```python
from build123d import *

# Parameters (mm, degrees)
EXTRUDE_1_DEPTH     = 2
SKETCH_2_W          = 6
SKETCH_2_H          = 12
EXTRUDE_2_DEPTH     = 5
FILLET_1_RADIUS     = 3
FILLET_1_LENGTH     = 10
SKETCH_4_R          = 1.1
CUT_EXTRUDE_2_DEPTH = 28
SKETCH_7_R          = 1.1
CUT_EXTRUDE_5_DEPTH = 3.5
SKETCH_9_R          = 1.5
CUT_EXTRUDE_7_DEPTH = 0.1
SKETCH_15_W         = 6
SKETCH_15_H         = 9.205828816
CUT_EXTRUDE_8_DEPTH = 10


with BuildPart() as part:
    # 草图1 → 凸台-拉伸1 (new body)
    with BuildSketch(Plane(origin=(0, 0, 0), x_dir=(1, 0, 0), z_dir=(0, 1, 0))):
        with BuildLine():
            Line((-7, 3), (7, 3))
            ThreePointArc((7, 3), (10, 0), (7, -3))
            Line((7, -3), (-7, -3))
            ThreePointArc((-7, -3), (-10, 0), (-7, 3))
        make_face()
    extrude(amount=EXTRUDE_1_DEPTH)

    # 草图2 → 凸台-拉伸2 (add, symmetric)
    with BuildSketch(Plane(origin=(0, 0, 0), x_dir=(0, 0, -1), z_dir=(1, 0, 0))):
        with Locations((0, 6)):
            Rectangle(SKETCH_2_W, SKETCH_2_H)
    extrude(amount=EXTRUDE_2_DEPTH, both=True)

    # 圆角1: full round fillet: the end face becomes a half cylinder, R = half its width
    fillet_1_face = Plane((0, 12, 0), x_dir=(1, 0, 0), z_dir=(0, 1, 0))  # on the end face: x along it, z out of the body
    fillet_1_slab = fillet_1_face.offset(-FILLET_1_RADIUS / 2) * Box(FILLET_1_LENGTH, 2 * FILLET_1_RADIUS, FILLET_1_RADIUS, mode=Mode.PRIVATE)  # the body's end, R deep
    fillet_1_round = Plane((0, 9, 0), x_dir=(0, 1, 0), z_dir=(1, 0, 0)) * Cylinder(FILLET_1_RADIUS, FILLET_1_LENGTH, mode=Mode.PRIVATE)  # its axis R under the face
    add(fillet_1_slab - fillet_1_round, mode=Mode.SUBTRACT)

    # 草图4 → 切除-拉伸2 (cut)
    with BuildSketch(Plane(origin=(5, 0, 0), x_dir=(0, 0, -1), z_dir=(1, 0, 0))):
        with Locations((0, 9)):
            Circle(SKETCH_4_R)
    extrude(amount=-CUT_EXTRUDE_2_DEPTH, mode=Mode.SUBTRACT)

    # 草图7 → 切除-拉伸5 (cut)
    with BuildSketch(Plane(origin=(0, 2, 0), x_dir=(1, 0, 0), z_dir=(0, 1, 0))):
        with Locations(Location((7, 0, 0), (0, 0, 270))):
            Circle(SKETCH_7_R)
        with Locations(Location((-7, 0, 0), (0, 0, 270))):
            Circle(SKETCH_7_R)
    extrude(amount=-CUT_EXTRUDE_5_DEPTH, mode=Mode.SUBTRACT)

    # 草图9 → 切除-拉伸7 (cut)
    with BuildSketch(Plane.XZ):
        with Locations(Location((0, 0, 0), (0, 0, 270))):
            Circle(SKETCH_9_R)
    extrude(amount=-CUT_EXTRUDE_7_DEPTH, mode=Mode.SUBTRACT)

    # 草图15 → 切除-拉伸8 (cut)
    with BuildSketch(Plane(origin=(0, 0, -3), x_dir=(-1, 0, 0), z_dir=(0, 0, -1))):
        with Locations((0, 9.102914408)):
            Rectangle(SKETCH_15_W, SKETCH_15_H)
    extrude(amount=-CUT_EXTRUDE_8_DEPTH, mode=Mode.SUBTRACT)


solid = part.part
```
Verification items for the finished model (mm, model axes). A direction names the side the tool comes from. Coordinates: 2 decimals unless noted, no trailing zeros. Order: outer loops, then holes, each group sorted by start corner. A loop starts at its lowest first (then second) coordinate and runs counter-clockwise, first axis right, second up. Notation, with made-up numbers: (-34.75, 25) - (-9.75, 25) arc R21 cw to (-9.75, 40) - close; hole circle Ø11 at (83, 12.25). An arc over 180 degrees is marked (long way). Return JSON: item names as keys, results as strings.
(1) Section check B-B, the plane z = 0. Give the number of separate pieces and of enclosed holes in the cut face, and give its area (3 significant figures).
Filled sheet:
{"separate pieces": "5", "enclosed holes": "0", "area": "77.1 mm^2"}
(2) Thickness scan on line 1 along X through (y, z) = (1.2, 0); line 2 along Y through (x, z) = (-4.25, 0.05); line 3 along X through (y, z) = (10.5, -2.4). Record the ranges inside material, lowest first.
Filled sheet:
{"line 1": "x = -10 to -8.1, -5.9 to 5.9, 8.1 to 10", "line 2": "y = 0 to 7.9, 10.1 to 12", "line 3": "x = -5 to -3, 3 to 5"}
(3) Section check D-D, the plane x = 6.75. Record the cut outline in (y, z), and give its area (3 significant figures).
Filled sheet:
{"outline": "(0, -3) - (2, -3) - (2, -1.07) - (0, -1.07) - close; (0, 1.07) - (2, 1.07) - (2, 3) - (0, 3) - close", "area": "7.72 mm^2"}
(4) Section check A-A, the plane y = 5. Record the cut outline in (x, z).
Filled sheet:
{"outline": "(-5, -3) - (-3, -3) - (-3, 3) - (-5, 3) - close; (3, -3) - (5, -3) - (5, 3) - (3, 3) - close"}
(5) Access from +Z, -Z, +X, -X, +Y, -Y to the whole of each face (thin tool, end or side, straight path). Record for faces 1 (the flat face through (0, 0.1, 0)), 2 (the flat face through (-8, 2, 1)), 3 (the flat face through (8, 2, 1)), 4 (the flat face through (3, 7, 0)), 5 (the cylindrical face through (-10, 1, 0)).
Filled sheet:
{"face 1": "-Y", "face 2": "+Z, -Z, -X, +Y", "face 3": "+Z, -Z, +X, +Y", "face 4": "+Z, -Z, +Y", "face 5": "-X, +Y, -Y"}
(6) Go/stop test with flat-tipped pins: pin 1 (1.8 mm diameter, centred on y = 10, z = 0, fed in from -X); pin 2 (2 mm diameter, centred on y = 9, z = 0, fed in from +X); pin 3 (1 mm diameter, centred on y = 6, z = 0, fed in from +X); pin 4 (1.5 mm diameter, centred on x = 4.5, z = -1.5, fed in from +Y). Record where each tip stops, or that it passes through.
Filled sheet:
{"pin 1": "stops at x = -5", "pin 2": "passes through", "pin 3": "stops at x = 5", "pin 4": "stops at y = 11.9"}
(7) Section check C-C, the plane y = 9.5. Record the cut outline in (x, z).
Filled sheet:
{"outline": "(-5, -2.96) - (-3, -2.96) - (-3, -0.98) - (-5, -0.98) - close; (-5, 0.98) - (-3, 0.98) - (-3, 2.96) - (-5, 2.96) - close; (3, -2.96) - (5, -2.96) - (5, -0.98) - (3, -0.98) - close; (3, 0.98) - (5, 0.98) - (5, 2.96) - (3, 2.96) - close"}
(8) Mould release check, pull along Z, two halves, no side actions. Record for faces 6 (the flat face through (0, 4.5, 0)), 7 (the cylindrical face through (-3.986, 7.926, 0.238)), 8 (the cylindrical face through (10, 1, 0)): pulls with the +Z half, pulls with the -Z half, needs draft (parallel to the pull), parting line crosses it, or undercut.
Filled sheet:
{"face 6": "needs draft", "face 7": "undercut", "face 8": "parting line crosses it"}
